Can you work these out from the drawing? Everything is in mm from the part's minimum corner. A direction names the side the tool comes from. Coordinates: 2 decimals unless noted, no trailing zeros. Order: outer loops, then holes, each group sorted by start corner. A loop starts at its lowest first (then second) coordinate and runs counter-clockwise, first axis right, second up. Notation, with made-up numbers: (-3, 34) - (16, 34) arc R24 ccw to (16, 50) - close; hole circle Ø9 at (89.5, 19.5). An arc over 180 degrees is marked (long way). Answer as CSV lines item,"result". Start each with the question number.
Q1. For pin 1 Ø6 at (x, y) = (13.5, 55) entering from -Z; pin 2 Ø3 at (y, z) = (61, 11) entering from -X, each with a flat end and sliding along its axis, tell me the tip position at first contact or that it passes through.
Q2. Suppose I cut it at B-B (x = 10). Please give me the cut outline in (y, z).
Q3. I need wall thicknesses on line 1 (Y direction, x = 10, z = 20.7); line 2 (Z direction, x = 13, y = 37). Which ranges of each line are inside material? Lowest first, please.
Q4. For the marked faces 1 and 2, which set-ups out of +Z, -Z, +X, -X, +Y, -Y let a thin tool reach every point of the face, with its end or its side?
Q5. Suppose I cut it at C-C (z = 8.25). Please give me the cut outline in (x, y).
Q6. Suppose I cut it at D-D (y = 16). Please give me the cut outline in (x, z), then the cut area to 3 significant figures.
Q7. Suppose I cut it at A-A (y = 50). Please give me the cut outline in (x, z), then the cut area to 3 significant figures.
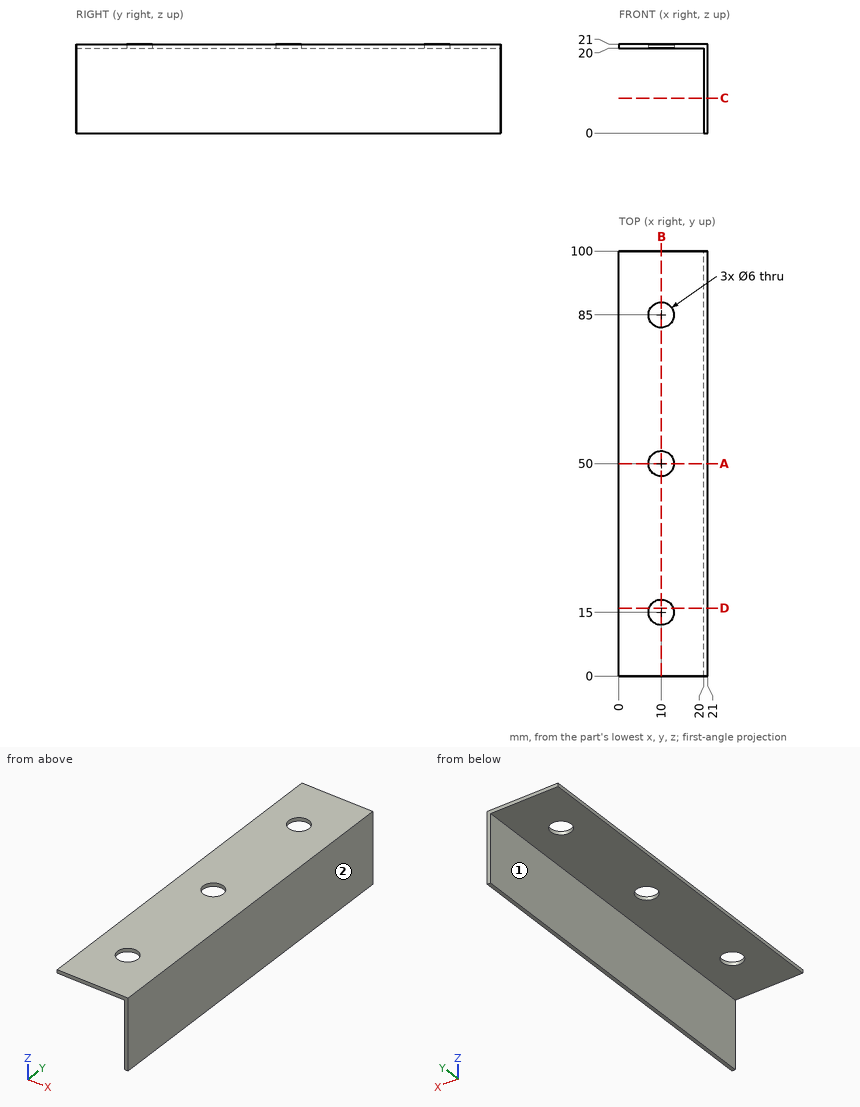
Here are the results:
1,pin 1,"stops at z = 20"
1,pin 2,"stops at x = 20"
2,outline,"(0, 20) - (12, 20) - (12, 21) - (0, 21) - close; (18, 20) - (47, 20) - (47, 21) - (18, 21) - close; (53, 20) - (82, 20) - (82, 21) - (53, 21) - close; (88, 20) - (100, 20) - (100, 21) - (88, 21) - close"
3,line 1,"y = 0 to 12, 18 to 47, 53 to 82, 88 to 100"
3,line 2,"z = 20 to 21"
4,face 1,"-Z, -X, +Y, -Y"
4,face 2,"+Z, -Z, +X, +Y, -Y"
5,outline,"(20, 0) - (21, 0) - (21, 100) - (20, 100) - close"
6,outline,"(0, 20) - (7.17, 20) - (7.17, 21) - (0, 21) - close; (12.83, 20) - (20, 20) - (20, 0) - (21, 0) - (21, 21) - (12.83, 21) - close"
6,area,"35.3 mm²"
7,outline,"(0, 20) - (7, 20) - (7, 21) - (0, 21) - close; (13, 20) - (20, 20) - (20, 0) - (21, 0) - (21, 21) - (13, 21) - close"
7,area,"35.0 mm²"
